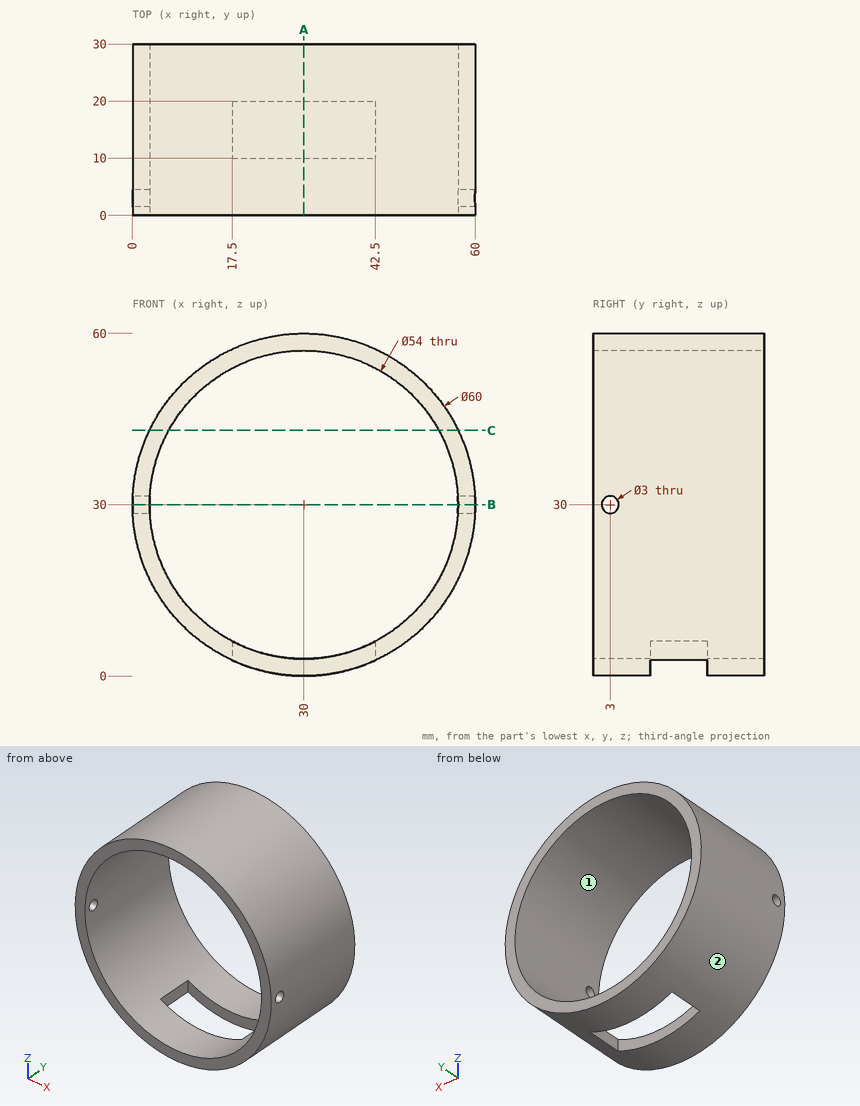
Source: three-view drawing plus pictorial views. Frame: mm from the lowest corner of the part. Round coordinates to 2 decimals unless told otherwise and drop trailing zeros. Loops run counter-clockwise (first coordinate to the right, second up) from the corner with the lowest first, then second, coordinate; pieces in that order, holes last. Notation, with made-up numbers: (-2.75, 24.25) - (1.25, 24.25) arc R30 cw to (1.25, 61.25) - close; hole circle Ø8 at (2.25, -12.75). An arc over 180 degrees is marked (long way). Write item = value, one per line. Start each with the question number.
Item 1: First-contact query: pin 1 Ø2 at (x, y) = (52.5, 18.5) entering from +Z; pin 2 Ø6 at (y, z) = (7, 41) entering from +X; pin 3 Ø8 at (y, z) = (22, 47) entering from +X; pin 4 Ø2.5 at (y, z) = (3, 30) entering from +X. Flat tips, straight axial feed; report the tip coordinate or a pass-through.
Item 2: Mould query, pull axis X, two halves, no side actions, for the marked faces 1 and 2. Classes: released by +X, released by -X, zero draft, split by the parting line, or undercut.
Item 3: Material intervals for line 1 (X direction, y = 11, z = 30); line 2 (Y direction, x = 1, z = 30); line 3 (Z direction, x = 49, y = 24), sorted ascending.
Item 4: Section query C-C on z = 43. Output: boundary loops of the cut face in (x, y), plus the area to 3 significant figures.
Item 5: Section query B-B on z = 30. Output: boundary loops of the cut face in (x, y), plus the area to 3 significant figures.
Item 6: Section query A-A on x = 30. Output: boundary loops of the cut face in (y, z), plus the area to 3 significant figures.
Results list:
q1.pin_1 = 50.92
q1.pin_2 = 58.91
q1.pin_3 = 57.04
q1.pin_4 = through
q2.face_1 = undercut
q2.face_2 = split by the parting line
q3.line_1 = 0 to 3, 57 to 60
q3.line_2 = 0 to 1.5, 4.5 to 30
q3.line_3 = 6.78 to 10.82, 49.18 to 53.22
q4.outline = (2.96, 0) - (6.34, 0) - (6.34, 30) - (2.96, 30) - close; (53.66, 0) - (57.04, 0) - (57.04, 30) - (53.66, 30) - close
q4.area = 202 mm²
q5.outline = (0, 0) - (3, 0) - (3, 1.5) - (0, 1.5) - close; (0, 4.5) - (3, 4.5) - (3, 30) - (0, 30) - close; (57, 0) - (60, 0) - (60, 1.5) - (57, 1.5) - close; (57, 4.5) - (60, 4.5) - (60, 30) - (57, 30) - close
q5.area = 162 mm²
q6.outline = (0, 0) - (10, 0) - (10, 3) - (0, 3) - close; (0, 57) - (30, 57) - (30, 60) - (0, 60) - close; (20, 0) - (30, 0) - (30, 3) - (20, 3) - close
q6.area = 150 mm²
